from build123d import *

# Parameters (mm, degrees)
FILLET1_R = 22
SHELL1_T  = -0.25


with BuildPart() as part:
    # Sketch1 → Revolve3 (revolve)
    with BuildSketch(Plane.XY, mode=Mode.PRIVATE) as revolve3_sk:
        Polygon((0, 0), (4.5, 0), (4.5, 4), (7, 4), (7, 4.5), (4.021373221, 5.618538642), (0, 6), align=None)
    revolve(revolve3_sk.sketch.rotate(Axis((0, 6, 0), (0, -1, 0)), 90), axis=Axis((0, 6, 0), (0, -1, 0)))

    # Fillet1
    fillet1_edges = [part.edges().sort_by_distance(p)[0] for p in [
        (0, 5.618538642, -4.021373221),
    ]]
    fillet(fillet1_edges, radius=FILLET1_R)

    # Shell1
    shell1_openings = [part.faces().sort_by_distance(p)[0] for p in [
        (0, 0, 0),
    ]]
    offset(amount=SHELL1_T, openings=shell1_openings, kind=Kind.INTERSECTION)


solid = part.part
Work out the finished part from the listing and answer in its coordinate system (mm). Give positions to 0.01 mm unless a question says otherwise; leave off trailing zeros. Write each loop counter-clockwise with the first axis right and the second up, starting at its lowest first coordinate (ties: lowest second). Pieces come first, ordered by that corner, then holes.
Q1. The part is cut by section A-A on y = 2.75. Give the vertices of the cut face in (x, z), and give its area (3 significant figures).
Answer:
outline: circle Ø9 at (0, 0); hole circle Ø8.5 at (0, 0)
area: 6.87 mm2
Q2. Straight lines are drawn through the part: L1, parallel to X at y = 1.2, z = 0; L2, parallel to X at y = 4.3, z = 0; L3, parallel to Z at x = -2.5, y = 1. For each, find the intervals that lie inside material, in ascending order.
Answer:
L1: x = -4.5 to -4.25, 4.25 to 4.5
L2: x = -7 to -6.75, 6.75 to 7
L3: z = -3.74 to -3.44, 3.44 to 3.74
Q3. Given pin 1 (2 mm diameter, centred on y = 3.5, z = 5, fed in from +X); pin 2 (1 mm diameter, centred on y = 3, z = 2, fed in from +X); pin 3 (4 mm diameter, centred on x = -1, z = 2.5, fed in from +Y), each flat-ended and moving along its own axis, determine where each tip first touches the part or whether it passes through.
Answer:
pin 1: stops at x = 5.65
pin 2: stops at x = 4.24
pin 3: stops at y = 5.93
Q4. For a pull along Y with two mould halves and no side action, classify faces 1 (the face through (-0.1, 4.25, -4.4)), 2 (the face through (0, 6, 0)), 3 (the face through (6.21, 4.25, 3.23)), 4 (the face through (0.02, 5.744, 0.049)) as released by +Y, released by -Y, zero draft, split by the parting line, or undercut.
Answer:
face 1: undercut
face 2: released by +Y
face 3: zero draft
face 4: released by -Y
